Answer from the drawing. Dimensions are ordinates in mm from the lowest x, y and z of the part. Round coordinates to 2 decimals unless told otherwise and drop trailing zeros. Order: outer loops, then holes, each group sorted by start corner. A loop starts at its lowest first (then second) coordinate and runs counter-clockwise, first axis right, second up. Notation, with made-up numbers: (-32, 29) -> (2, 29) arc R28 ccw to (2, 59) -> close; hole circle Ø2 at (43, 89). An arc over 180 degrees is marked (long way). Use a Markdown table: item, result. Add a question column.
1. Section B-B, the plane y = 7 is taken. Give the vertices of the cut face in (x, z) (1 decimal).
2. Given pin 1 (1.5 mm diameter, centred on x = 37, z = 1.5, fed in from -Y); pin 2 (1.5 mm diameter, centred on x = 59.5, z = 2.5, fed in from -Y); pin 3 (1 mm diameter, centred on y = 49.5, z = 1.5, fed in from -X) (1 decimal), each flat-ended and moving along its own axis, determine where each tip first touches the part or whether it passes through.
3. Section A-A, the plane z = 1.45 is taken. Give the vertices of the cut face in (x, y) (1 decimal), then the cut area to 3 significant figures.
4. Section C-C, the plane x = 66 is taken. Give the vertices of the cut face in (y, z).
5. Consider L1, parallel to Y at x = 53, z = 0.2; L2, parallel to Y at x = 99.5, z = 0.65; L3, parallel to X at y = 53, z = 0.5. Determine where each line is inside the solid, lowest interval first. Write a range as [from, to].
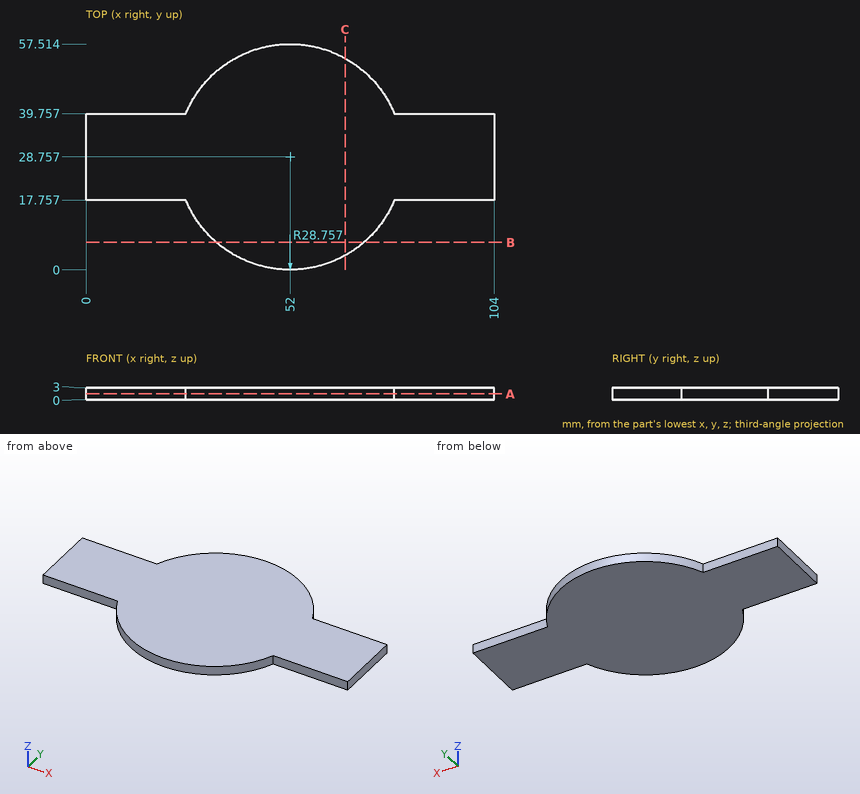
Verdict:
| question | item | result |
|---|---|---|
| 1 | outline | (33.2, 0) -> (70.8, 0) -> (70.8, 3) -> (33.2, 3) -> close |
| 2 | pin 1 | stops at y = 3.78 |
| 2 | pin 2 | stops at y = 0.8 |
| 2 | pin 3 | stops at x = 31.6 |
| 3 | outline | (0, 17.8) -> (25.4, 17.8) arc R28.8 ccw to (78.6, 17.8) -> (104, 17.8) -> (104, 39.8) -> (78.6, 39.8) arc R28.8 ccw to (25.4, 39.8) -> (0, 39.8) -> close |
| 3 | area | 3,650 mm2 |
| 4 | outline | (3.64, 0) -> (53.88, 0) -> (53.88, 3) -> (3.64, 3) -> close |
| 5 | L1 | y = [0.02, 57.5] |
| 5 | L2 | y = [17.76, 39.76] |
| 5 | L3 | x = [36.53, 67.47] |
